The listing builds one solid part. Answer for the finished solid, in the listing's coordinates (mm). Round coordinates to 2 decimals unless told otherwise and drop trailing zeros. Order: outer loops, then holes, each group sorted by start corner. A loop starts at its lowest first (then second) coordinate and runs counter-clockwise, first axis right, second up. Notation, with made-up numbers: M 88.5,-24 L 113.5,-24 A21 ccw 113.5,8 Z; hole C 56.5,9.25 d3. An arc over 180 degrees is marked long. Write item = value, one per line. Start each with the question number.
(1) A cutting plane is placed at A-A, the plane y = 0.7. Determine the outline of the cut face in (x, z), and give its area (3 significant figures).
(2) A cutting plane is placed at D-D, the plane x = 0.15. Determine the outline of the cut face in (y, z), and give its area (3 significant figures).
(3) Straight lines are drawn through the part: probe 1 along Z at (x, y) = (0.2, 0.8); probe 2 along X at (y, z) = (0.75, -4.5); probe 3 along Z at (x, y) = (0.8, 1.2). For each, find the intervals that lie inside material, in ascending order. Write a range as from..to.
(4) A cutting plane is placed at C-C, the plane x = 0.8. Determine the outline of the cut face in (y, z), and give its area (3 significant figures).
(5) A cutting plane is placed at B-B, the plane z = 4. Determine the outline of the cut face in (x, y).
from build123d import *

# Parameters (mm, degrees)
SKETCH1_W           = 4
SKETCH1_H           = 16.1
BOSS_EXTRUDE1_DEPTH = 1.45
SKETCH2_W           = 2.0696
SKETCH2_H           = 15.084
CUT_EXTRUDE1_DEPTH  = 1
SKETCH3_W           = 1.143
SKETCH3_H           = 12.798
BOSS_EXTRUDE2_DEPTH = 1


with BuildPart() as part:
    # Sketch1 → Boss-Extrude1 (new body)
    with BuildSketch(Plane(origin=(0, 1.45, 0), x_dir=(-1, 0, 0), z_dir=(0, 1, 0))):
        Rectangle(SKETCH1_W, SKETCH1_H)
    extrude(amount=-BOSS_EXTRUDE1_DEPTH)

    # Sketch2 → Cut-Extrude1 (cut)
    with BuildSketch(Plane(origin=(0, 1.45, 0), x_dir=(-1, 0, 0), z_dir=(0, 1, 0))):
        Rectangle(SKETCH2_W, SKETCH2_H)
    extrude(amount=-CUT_EXTRUDE1_DEPTH, mode=Mode.SUBTRACT)

    # Sketch3 → Boss-Extrude2 (add)
    with BuildSketch(Plane(origin=(0, 0.45, 0), x_dir=(-1, 0, 0), z_dir=(0, 1, 0))):
        Rectangle(SKETCH3_W, SKETCH3_H)
    extrude(amount=BOSS_EXTRUDE2_DEPTH)


solid = part.part
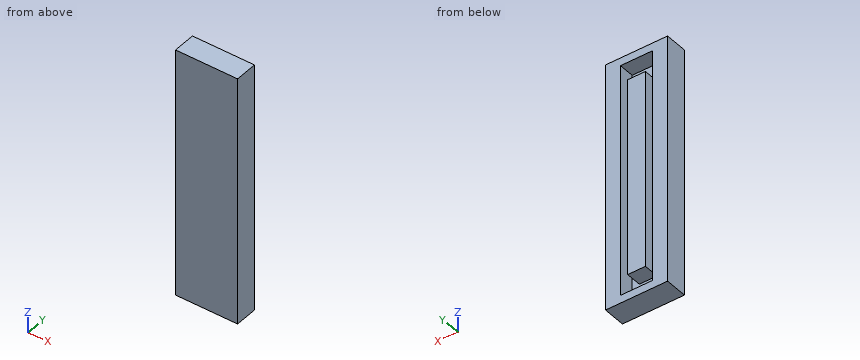
Reported:
q1.outline = M -2,-8.05 L 2,-8.05 L 2,8.05 L -2,8.05 Z; M -0.57,-6.4 L 0.57,-6.4 L 0.57,6.4 L -0.57,6.4 Z; hole M -1.03,-7.54 L 1.03,-7.54 L 1.03,7.54 L -1.03,7.54 Z
q1.area = 47.8 mm²
q2.outline = M 0,-8.05 L 1.45,-8.05 L 1.45,-7.54 L 0.45,-7.54 L 0.45,-6.4 L 1.45,-6.4 L 1.45,6.4 L 0.45,6.4 L 0.45,7.54 L 1.45,7.54 L 1.45,8.05 L 0,8.05 Z
q2.area = 21.1 mm²
q3.probe_1 = -8.05..-7.54, -6.4..6.4, 7.54..8.05
q3.probe_2 = -2..-1.03, -0.57..0.57, 1.03..2
q3.probe_3 = -8.05..-7.54, 7.54..8.05
q4.outline = M 0,-8.05 L 1.45,-8.05 L 1.45,-7.54 L 0.45,-7.54 L 0.45,7.54 L 1.45,7.54 L 1.45,8.05 L 0,8.05 Z
q4.area = 8.26 mm²
q5.outline = M -2,0 L 2,0 L 2,1.45 L 1.03,1.45 L 1.03,0.45 L 0.57,0.45 L 0.57,1.45 L -0.57,1.45 L -0.57,0.45 L -1.03,0.45 L -1.03,1.45 L -2,1.45 Z
